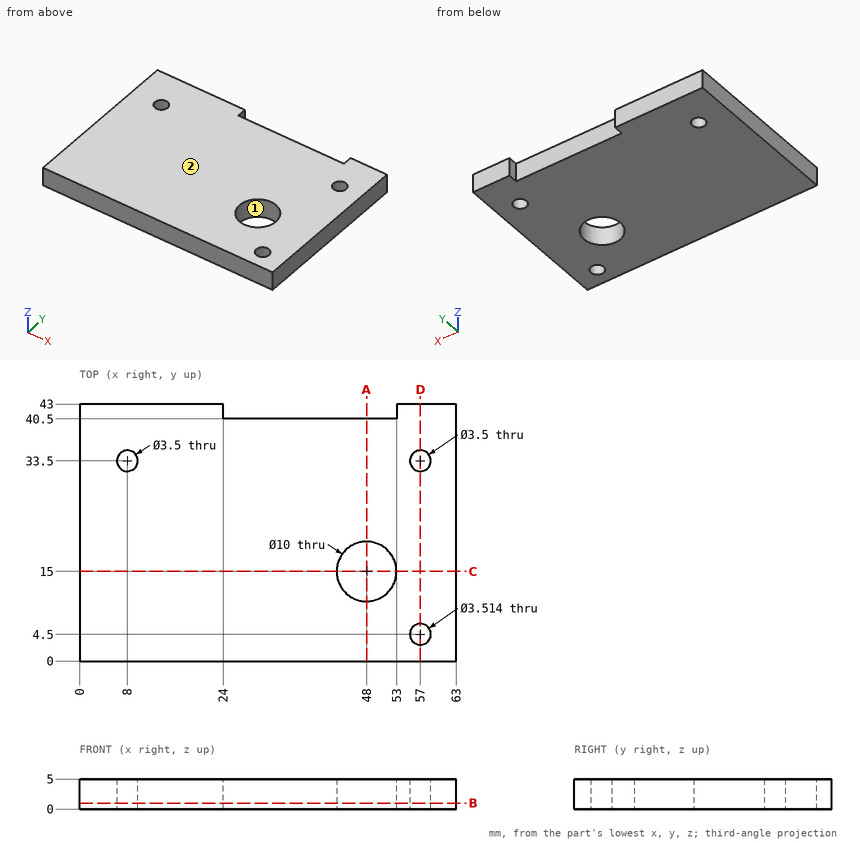
Input: dimensioned drawing with shaded views. Units: mm. Origin: part minimum x, y, z. Coordinates: 2 decimals unless noted, no trailing zeros. Order: outer loops, then holes, each group sorted by start corner. A loop starts at its lowest first (then second) coordinate and runs counter-clockwise, first axis right, second up.
1. Cut plane A-A, the plane x = 48. Return loops of the section in (y, z).
Checked values:
outline: (0, 0) - (10, 0) - (10, 5) - (0, 5) - close; (20, 0) - (40.5, 0) - (40.5, 5) - (20, 5) - close
2. Draft query along Y for the marked faces 1 and 2. Return one class per face: +Y half, -Y half, draft (parallel to the pull), parting line (faces both ways), or undercut.
Checked values:
face 1: undercut
face 2: draft
3. Cut plane C-C, the plane y = 15. Return loops of the section in (x, z), plus the area to 3 significant figures.
Checked values:
outline: (0, 0) - (43, 0) - (43, 5) - (0, 5) - close; (53, 0) - (63, 0) - (63, 5) - (53, 5) - close
area: 265 mm2
4. Cut plane D-D, the plane x = 57. Return loops of the section in (y, z), plus the area to 3 significant figures.
Checked values:
outline: (0, 0) - (2.74, 0) - (2.74, 5) - (0, 5) - close; (6.26, 0) - (31.75, 0) - (31.75, 5) - (6.26, 5) - close; (35.25, 0) - (43, 0) - (43, 5) - (35.25, 5) - close
area: 180 mm2
5. Ray query, line 1 along Y through (x, z) = (57, 1.6); line 2 along Y through (x, z) = (58, 4.8) (1 decimal); line 3 along X through (y, z) = (41, 3.1). Return the intervals inside material, ascending.
Checked values:
line 1: y = 0 to 2.74, 6.26 to 31.75, 35.25 to 43
line 2: y = 0 to 3.1, 5.9 to 32.1, 34.9 to 43
line 3: x = 0 to 24, 53 to 63
6. Contact query for flat-ended pins moving along their axis: P1, Ø3, axis at x = 57, y = 33.5, coming from the +Z side; P2, Ø2, axis at x = 49.5, z = 1.5, coming from the +Y side. Output: stop coordinate, or through.
Checked values:
P1: passes through
P2: stops at y = 40.5
7. Cut plane B-B, the plane z = 1. Return loops of the section in (x, y).
Checked values:
outline: (0, 0) - (63, 0) - (63, 43) - (53, 43) - (53, 40.5) - (24, 40.5) - (24, 43) - (0, 43) - close; hole circle Ø3.5 at (8, 33.5); hole circle Ø10 at (48, 15); hole circle Ø3.51 at (57, 4.5); hole circle Ø3.5 at (57, 33.5)
